```python
from build123d import *

# Parameters (mm, degrees)
F0_R      = 5.5
F1_DEPTH  = 12
F2_W      = 12
F2_H      = 76
F3_DEPTH  = 50
F4_R      = 5.5
F5_DEPTH  = 12
F8_R      = 19
F6_R      = 24
F10_R     = 10
F11_DEPTH = 46
F13_DEPTH = 76


with BuildPart() as f1:
    # F0 (on Right) → F1 (new body)
    with BuildSketch(Plane.YZ):
        with BuildLine():
            ThreePointArc((0, 12), (3.5147186258, 3.5147186258), (12, 0))
            Line((12, 0), (100, 0))
            Line((100, 0), (100, 76))
            Line((100, 76), (12, 76))
            ThreePointArc((12, 76), (3.5147186258, 72.4852813742), (0, 64))
            Line((0, 64), (0, 12))
        make_face()
        with Locations((12, 12)):
            Circle(F0_R, mode=Mode.SUBTRACT)
        with Locations((12, 64)):
            Circle(F0_R, mode=Mode.SUBTRACT)
    extrude(amount=F1_DEPTH)

    # F2 (on face) → F3 (join)
    with BuildSketch(Plane.YZ.offset(12)):
        with Locations((94, 38)):
            Rectangle(F2_W, F2_H)
    extrude(amount=F3_DEPTH)

    # F4 (on face) → F5 (cut)
    with BuildSketch(Plane.XZ.offset(-88)):
        with Locations((32, 64)):
            Circle(F4_R)
        with Locations((32, 12)):
            Circle(F4_R)
        with BuildLine():
            ThreePointArc((50, 76), (58.4852813742, 72.4852813742), (62, 64))
            Line((62, 64), (62, 76))
            Line((62, 76), (50, 76))
        make_face()
        with BuildLine():
            Line((62, 0), (62, 12))
            ThreePointArc((62, 12), (58.4852813742, 3.5147186258), (50, 0))
            Line((50, 0), (62, 0))
        make_face()
    extrude(amount=-F5_DEPTH, mode=Mode.SUBTRACT)

    # F8 (on offset) → F9 section 0
    with BuildSketch(Plane.YZ.offset(46)):
        with Locations((50, 38)):
            Circle(F8_R)
    # F6 (on face) → F9 section 1
    with BuildSketch(Plane.YZ.offset(12)):
        with Locations((50, 38)):
            Circle(F6_R)
    loft()

    # F10 (on face) → F11 (cut)
    with BuildSketch(Plane.YZ.offset(46)):
        with Locations((50, 38)):
            Circle(F10_R)
    extrude(amount=-F11_DEPTH, mode=Mode.SUBTRACT)

    # F12 (on face) → F13 (join)
    with BuildSketch(Plane.XY.offset(76)):
        with BuildLine():
            ThreePointArc((12, 84), (13.1715728753, 86.8284271247), (16, 88))
            Line((16, 88), (12, 88))
            Line((12, 88), (12, 84))
        make_face()
    extrude(amount=-F13_DEPTH)


solid = f1.part
```
Work out the finished part from the listing and answer in its coordinate system (mm). A direction names the side the tool comes from. Coordinates: 2 decimals unless noted, no trailing zeros. Write each loop counter-clockwise with the first axis right and the second up, starting at its lowest first coordinate (ties: lowest second). Pieces come first, ordered by that corner, then holes. Notation, with made-up numbers: (-16, 40.25) - (33, 40.25) arc R27 cw to (33, 79.25) - close; hole circle Ø4 at (12.5, 69). An arc over 180 degrees is marked (long way). Answer as a JSON object with one key per item and string values.
Q1. Find section C-C (x = 6.5). Write down the section's boundary in (y, z), plus the area to 3 significant figures.
Results list:
{"outline": "(0, 12) arc R12 ccw to (12, 0) - (100, 0) - (100, 76) - (12, 76) arc R12 ccw to (0, 64) - close; hole circle Ø11 at (12, 12); hole circle Ø11 at (12, 64); hole circle Ø20 at (50, 38)", "area": "7,030 mm^2"}
Q2. Which of the six approach directions +Z, -Z, +X, -X, +Y, -Y give full straight-line access (tool end or side, diameter ignored) to faces 1 (the flat face through (46, 58, 30)), 2 (the flat face through (62, 94, 38)), 3 (the flat face through (39, 88, 37))?
Results list:
{"face 1": "+Z, -Z, +X, -Y", "face 2": "+Z, -Z, +X, +Y, -Y", "face 3": "+Z, -Z, +X"}
Q3. Consider L1, parallel to Z at x = 8, y = 12; L2, parallel to X at y = 51.5, z = 64; L3, parallel to Y at x = 55, z = 12. Determine where each line is inside the solid, lowest interval first. Write a range as from..to.
Results list:
{"L1": "z = 0..6.5, 17.5..58.5, 69.5..76", "L2": "x = 0..12", "L3": "y = 88..100"}
Q4. Given pin 1 Ø5 at (x, z) = (50, 58) entering from -Y; pin 2 Ø10 at (x, y) = (41, 79) entering from +Z; pin 3 Ø12.5 at (y, z) = (12, 12) entering from +X; pin 4 Ø10 at (y, z) = (23, 11) entering from -X, each flat-ended and moving along its own axis, determine where each tip first touches the part or whether it passes through.
Results list:
{"pin 1": "stops at y = 88", "pin 2": "passes through", "pin 3": "stops at x = 12", "pin 4": "stops at x = 0"}
Q5. For a pull along Z with two mould halves and no side action, classify faces 4 (the flat face through (10, 63, 76)), 5 (the flat face through (12, 23, 39)), 6 (the cylindrical face through (5.92, 3.42, 3.61)), 7 (the cylindrical face through (27.6, 93.9, 8.7)) as pulls with the +Z half, pulls with the -Z half, needs draft (parallel to the pull), parting line crosses it, or undercut.
Results list:
{"face 4": "pulls with the +Z half", "face 5": "needs draft", "face 6": "pulls with the -Z half", "face 7": "undercut"}
Q6. Find section D-D (x = 20). Write down the section's boundary in (y, z), plus the area to 3 significant figures.
Results list:
{"outline": "circle Ø45.65 at (50, 38); (88, 0) - (100, 0) - (100, 76) - (88, 76) - close; hole circle Ø20 at (50, 38)", "area": "2,230 mm^2"}
Q7. Find section A-A (y = 50). Write down the section's boundary in (x, z), plus the area to 3 significant figures.
Results list:
{"outline": "(0, 0) - (12, 0) - (12, 14) - (46, 19) - (46, 28) - (0, 28) - close; (0, 48) - (46, 48) - (46, 57) - (12, 62) - (12, 76) - (0, 76) - close", "area": "1,450 mm^2"}
Q8. Find section B-B (x = 33). Write down the section's boundary in (y, z), plus the area to 3 significant figures.
Results list:
{"outline": "circle Ø41.82 at (50, 38); (88, 0) - (100, 0) - (100, 6.59) - (88, 6.59) - close; (88, 17.41) - (100, 17.41) - (100, 58.59) - (88, 58.59) - close; (88, 69.41) - (100, 69.41) - (100, 76) - (88, 76) - close; hole circle Ø20 at (50, 38)", "area": "1,710 mm^2"}
